```python
from build123d import *

# Parameters (mm, degrees)
F4_DEPTH = 30


with BuildPart() as f3:
    # F0 (on Top) → F3 section 0
    with BuildSketch(Plane.XY):
        Polygon((-36.3730669589, -21), (0, -42), (36.3730669589, -21), (36.3730669589, 21), (0, 42), (-36.3730669589, 21), align=None)
    # F2 (on offset) → F3 section 1
    with BuildSketch(Plane.XY.offset(30)):
        Polygon((-51.9615242271, -30), (0, -60), (51.9615242271, -30), (51.9615242271, 30), (0, 60), (-51.9615242271, 30), align=None)
    loft()

    # F4 (add): a face of the model
    f4_faces = [f3.faces().sort_by_distance(p)[0] for p in [
        (0, 0, 30),
    ]]
    extrude(f4_faces, amount=F4_DEPTH)


solid = f3.part
```
The listing builds one solid part. Answer for the finished solid, in the listing's coordinates (mm). Coordinates: 2 decimals unless noted, no trailing zeros. Write each loop counter-clockwise with the first axis right and the second up, starting at its lowest first coordinate (ties: lowest second). Pieces come first, ordered by that corner, then holes. Notation, with made-up numbers: (49, 25) - (80, 25) arc R21 ccw to (80, 32) - close; hole circle Ø1 at (-25.75, 71). An arc over 180 degrees is marked (long way). Return JSON: item names as keys, results as strings. Group by question number.
1. Straight lines are drawn through the part: L1, parallel to Y at x = 29, z = 55.5; L2, parallel to X at y = -17.5, z = 27; L3, parallel to X at y = 36, z = 7.5. For each, find the intervals that lie inside material, in ascending order.
2. A cutting plane is placed at A-A, the plane z = 43. Determine the outline of the cut face in (x, y).
3. Given pin 1 (8 mm diameter, centred on y = 46, z = 28.5, fed in from -X); pin 2 (3 mm diameter, centred on x = -5.5, z = 18, fed in from +Y); pin 3 (3 mm diameter, centred on y = 17, z = 22.5, fed in from -X), each flat-ended and moving along its own axis, determine where each tip first touches the part or whether it passes through.
Ans:
{
 "1": {"L1": "-43.26 to 43.26", "L2": "-50.4 to 50.4", "L3": "-18.19 to 18.19"},
 "2": {"outline": "(-51.96, -30) - (0, -60) - (51.96, -30) - (51.96, 30) - (0, 60) - (-51.96, 30) - close"},
 "3": {"pin 1": "x = -30.67", "pin 2": "y = 50.87", "pin 3": "x = -48.84"}
}
